Check sheet for the modelled part. Datum: model origin and axes. Units: mm. A direction names the side the tool comes from. Give positions to 0.01 mm unless a question says otherwise; leave off trailing zeros. Loops run counter-clockwise (first coordinate to the right, second up) from the corner with the lowest first, then second, coordinate; pieces in that order, holes last.
Autodesk Inventor part; units mm, degrees
ref_plane "YZ Plane" through (0, 0, 0) normal (1, 0, 0) x (0, 1, 0)
ref_plane "XZ Plane" through (0, 0, 0) normal (0, 1, 0) x (-1, 0, 0)
ref_plane "XY Plane" through (0, 0, 0) normal (0, 0, 1) x (1, 0, 0)
sketch "Sketch3" plane through (0, 0, 0) normal (0, 0, 1) x (1, 0, 0)
  line L0 (-10.1, 25) -> (10.1, 25)
  line L1 (10.1, 25) -> (10.1, -25)
  line L2 (10.1, -25) -> (-10.1, -25)
  line L3 (-10.1, -25) -> (-10.1, 25)
  point P0 (0, 0)
  dimension "d26" = 20.2
  dimension "d27" = 50
extrude "Extrusion3" add sketch "Sketch3" along normal blind 1.8
sketch "Sketch4" plane through (0, 0, 1.8) normal (0, 0, 1) x (1, 0, 0)
  line L0 (-8.1, 23) -> (8.1, 23)
  line L1 (8.1, -23) -> (-8.1, -23)
  line L2 (-8.1, 0) -> (-8.1, 2.5)
  line L3 (-8.1, 2.5) -> (8.1, 2.5)
  line L4 (8.1, 4.5) -> (-8.1, 4.5)
  line L5 (-8.1, 0) -> (-8.1, -2.5)
  line L6 (-8.1, -2.5) -> (8.1, -2.5)
  line L7 (8.1, -4.5) -> (-8.1, -4.5)
  line L8 (-8.1, 4.5) -> (-8.1, 23)
  line L9 (8.1, 23) -> (8.1, 4.5)
  line L10 (8.1, 2.5) -> (8.1, -2.5)
  line L11 (8.1, -4.5) -> (8.1, -23)
  line L12 (-10.1, 25) -> (-10.1, -25)
  line L13 (10.1, -25) -> (10.1, 25)
  line L14 (-10.1, 25) -> (10.1, 25)
  line L15 (10.1, 25) -> (10.1, -25)
  line L16 (10.1, -25) -> (-10.1, -25)
  line L17 (-10.1, -25) -> (-10.1, 25)
  line L18 (-8.1, -23) -> (-8.1, -4.5)
  line L19 (-8.1, -2.5) -> (-8.1, 2.5)
  point P0 (0, 0)
  dimension "d39" = 2.5
  dimension "d40" = 2.5
  dimension "d44" = 2
  dimension "d45" = 2
  dimension "d48" = 2
  dimension "d49" = 2
  dimension "d50" = 2
  dimension "d51" = 2
  dimension "d52" = 2
  dimension "d53" = 2
  dimension "d56" = 2
  dimension "d57" = 2
extrude "Extrusion4" add sketch "Sketch4" along normal blind 8.2
sketch "Sketch5" plane through (10.1, -25, 0) normal (1, 0, 0) x (0, 0, -1)
  line L0 (-1.8, 27.5) -> (-10, 27.5)
  line L1 (-1.8, 22.5) -> (-10, 22.5)
  line L2 (-10, 27.5) -> (-1.8, 27.5)
  line L3 (-1.8, 27.5) -> (-1.8, 22.5)
  line L4 (-1.8, 22.5) -> (-10, 22.5)
  line L5 (-10, 22.5) -> (-10, 27.5)
  point P0 (0, 25)
extrude "Extrusion5" cut sketch "Sketch5" against normal blind 8.2
sketch "Sketch6" plane through (-10.1, -25, 0) normal (-1, 0, 0) x (0, 0, 1)
  line L0 (1.8, 27.5) -> (1.8, 22.5)
  line L1 (1.8, 22.5) -> (6.8, 22.5)
  line L2 (6.8, 22.5) -> (6.8, 27.5)
  line L3 (6.8, 27.5) -> (1.8, 27.5)
  line L4 (1.8, 27.5) -> (1.8, 22.5)
  point P0 (0, 25)
  dimension "d60" = 5
  dimension "d61" = 5
extrude "Extrusion6" cut sketch "Sketch6" against normal blind 8.2
sketch "Sketch7" plane through (-10.1, -25, 0) normal (-1, 0, 0) x (0, 0, 1)
  line L0 (0, 50) -> (10, 50)
  line L1 (0, 0) -> (0, 50)
  line L2 (0, 25) -> (10, 25)
  line L3 (0, 0) -> (10, 0)
  circle A0 centre (6.8, 45) radius 2
  circle A1 centre (8, 33) radius 2
  circle A2 centre (8, 17) radius 2
  circle A3 centre (6.8, 5) radius 2
  line L4 (6.8, 7) -> (10, 7)
  line L5 (6.8, 3) -> (10, 3)
  line L6 (10, 50) -> (10, 0)
  line L7 (10, 7) -> (10, 3)
  line L8 (6.8, 47) -> (10, 47)
  line L9 (10, 47) -> (10, 43)
  line L10 (10, 43) -> (6.8, 43)
  line L11 (10, 29.5) -> (10, 48)
  line L12 (8, 35) -> (10, 35)
  line L13 (10, 35) -> (10, 31)
  line L14 (10, 31) -> (8, 31)
  line L15 (8, 31) -> (8, 35)
  line L16 (10, 20.5) -> (10, 2)
  line L17 (8, 19) -> (10, 19)
  line L18 (10, 19) -> (10, 15)
  line L19 (10, 15) -> (8, 15)
  line L20 (8, 15) -> (8, 19)
  point P0 (4.5, 40)
  point P1 (4.5, 10)
  dimension "d66" = 10
  dimension "d67" = 4.5
  dimension "d70" = 5
  dimension "d71" = 6.8
  dimension "d74" = 17
  dimension "d75" = 8
  dimension "d90" = 4
  dimension "d91" = 4
hole "Hole1" at (-10.1, 15, 4.5) at (-10.1, -15, 4.5) direction (1, 0, 0) diameter 2.6 depth 2 tip angle 118
extrude "Extrusion7" cut sketch "Sketch7" against normal blind 2 contours L6 L10 A0 L8 | A0 | L14 A1 L6 | L6 A2 L17 | L6 A1 L12 | L5 A3 L4 L6 | A1 L15 | A1 L15 | A2 L20 | L6 L19 A2 | L20 A2 | A3
sketch "Sketch8" plane through (10.1, -25, 0) normal (1, 0, 0) x (0, 0, -1)
  line L0 (0, 50) -> (-10, 50)
  circle A0 centre (-6, 40) radius 2
  circle A1 centre (-6, 10) radius 2
  line L1 (-10, 15) -> (-10, 7)
  line L2 (-6, 12) -> (-10, 12)
  line L3 (-10, 12) -> (-10, 8)
  line L4 (-10, 8) -> (-6, 8)
  line L5 (-6, 8) -> (-6, 12)
  line L6 (-10, 43) -> (-10, 35)
  line L7 (-6, 42) -> (-10, 42)
  line L8 (-10, 42) -> (-10, 38)
  line L9 (-10, 38) -> (-6, 38)
  line L10 (-6, 38) -> (-6, 42)
  point P0 (0, 25)
  point P1 (-4.8, 45)
  point P2 (-6, 33)
  point P3 (-4.8, 5)
  point P4 (-6, 17)
  dimension "d113" = 4
  dimension "d114" = 4
hole "Hole3" at (10.1, 20, 4.8) at (10.1, -20, 4.8) direction (-1, 0, 0) diameter 2.6 depth 2 tip angle 118
hole "Hole4" at (10.1, 8, 6) at (10.1, -8, 6) direction (-1, 0, 0) diameter 3.6 depth 2 tip angle 118
extrude "Extrusion8" cut sketch "Sketch8" against normal blind 2
chamfer "Chamfer1" distance 1 angle 45 12 edges at (-9.1, 22, 10) (-9.1, 18, 10) (-9.1, 10, 10) (-9.1, 6, 10) (-9.1, -6, 10) (-9.1, -10, 10) (-9.1, -18, 10) (-9.1, -22, 10) (9.1, -17, 10) (9.1, -13, 10) (9.1, 13, 10) (9.1, 17, 10)
chamfer "Chamfer3" distance 1 angle 45 4 edges at (8.1, 20, 6.1) (8.1, -20, 6.1) (-8.1, -15, 3.2) (-8.1, 15, 3.2)
properties part number "digit_holder_B_no_hole"
(1) Section check A-A on y = -20. Record the boundary of the cut face in (x, z), plus the area to 3 significant figures.
(2) Gauge pin test, flat ends, axial feed: pin 1 Ø8 at (x, y) = (-3.5, 18.5) entering from +Z; pin 2 Ø2.5 at (y, z) = (-20, 4.8) entering from +X. Record the tip position at first contact, or that the pin passes through.
(3) Section check C-C on x = -3. Record the boundary of the cut face in (y, z), plus the area to 3 significant figures.
(4) Material ranges on line 1 (Y direction, x = -2, z = 3.5); line 2 (X direction, y = 10.5, z = 2.5); line 3 (Y direction, x = -9.8, z = 4.5), recorded low to high.
(5) Release check for a two-part mould opening along X. For faces 1 (the face through (-9.1, -22.5, 9.5)), 2 (the face through (-8.1, 0, 8)), 3 (the face through (0, 4.5, 6)) record: pulls with the +X half, pulls with the -X half, needs draft (parallel to the pull), parting line crosses it, or undercut.
(6) Section check D-D on y = 15. Record the boundary of the cut face in (x, z), plus the area to 3 significant figures.
(7) Section check B-B on y = -5.5. Record the boundary of the cut face in (x, z), plus the area to 3 significant figures.
(8) Access from +Z, -Z, +X, -X, +Y, -Y to the whole of each face (thin tool, end or side, straight path). Record for faces 4 (the face through (-9.1, 10, 8.5)), 5 (the face through (9.1, -12.5, 9.5)), 6 (the face through (0, -23, 6)), 7 (the face through (9.086, -6.403, 5.169)).
Computed values:
1. outline: (-10.1, 0) - (10.1, 0) - (10.1, 3.5) - (9.1, 3.5) - (8.1, 2.5) - (8.1, 1.8) - (-8.1, 1.8) - (-8.1, 4.8) - (-10.1, 4.8) - close; (8.1, 7.1) - (9.1, 6.1) - (10.1, 6.1) - (10.1, 10) - (8.1, 10) - close
1. area: 52.6 mm2
2. pin 1: stops at z = 1.8
2. pin 2: stops at x = -8.1
3. outline: (-25, 0) - (25, 0) - (25, 10) - (23, 10) - (23, 1.8) - (4.5, 1.8) - (4.5, 10) - (2.5, 10) - (2.5, 1.8) - (-2.5, 1.8) - (-2.5, 10) - (-4.5, 10) - (-4.5, 1.8) - (-23, 1.8) - (-23, 10) - (-25, 10) - close
3. area: 156 mm2
4. line 1: y = -25 to -23, -4.5 to -2.5, 2.5 to 4.5, 23 to 25
4. line 2: x = -10.1 to -8.1, 8.1 to 10.1
4. line 3: y = -25 to -16.3, -13.7 to -2.5, 2.5 to 13.7, 16.3 to 25
5. face 1: needs draft
5. face 2: pulls with the +X half
5. face 3: undercut
6. outline: (-10.1, 0) - (10.1, 0) - (10.1, 4) - (8.1, 4) - (8.1, 1.8) - (-8.1, 1.8) - (-8.1, 2.2) - (-9.1, 3.2) - (-10.1, 3.2) - close; (-10.1, 5.8) - (-9.1, 5.8) - (-8.1, 6.8) - (-8.1, 10) - (-10.1, 10) - close
6. area: 51.0 mm2
7. outline: (-10.1, 0) - (10.1, 0) - (10.1, 10) - (8.1, 10) - (8.1, 1.8) - (-8.1, 1.8) - (-8.1, 9.5) - (-10.1, 9.5) - close
7. area: 68.2 mm2
8. face 4: +Z, -X
8. face 5: +Z, +X
8. face 6: +Z
8. face 7: +X
